```python
from build123d import *

# Parameters (mm, degrees)
SKETCH_1_W                      = 7.778385112
SKETCH_1_H                      = 31.92137072
EXTRUDE_1_DEPTH                 = 8
SKETCH_2_R                      = 1.5
SKETCH_2_R_2                    = 2
CUT_EXTRUDE_1_DEPTH             = 8
SKETCH_3_W                      = 7.778385112
SKETCH_3_H                      = 11.681320089
CUT_EXTRUDE_2_DEPTH             = 7
CUT_EXTRUDE_3_DEPTH             = 7.778385113
CUT_EXTRUDE_6_REACH             = 24.375
CUT_EXTRUDE_7_DEPTH             = 1.25
CUT_EXTRUDE_7_DEPTH_BACK        = 1.25
CUT_EXTRUDE_8_REACH             = 24.375
SKETCH_8_R                      = 1
PATTERN_CIRCULAR_5_COUNT        = 2
CUT_EXTRUDE_9_DEPTH             = 23.991982407
CUT_EXTRUDE_9_DEPTH_BACK        = 23.991982407
PATTERN_START                   = 3.938890695
PATTERN_CIRCULAR_14_OUTLINE_R   = 1
PATTERN_CIRCULAR_14_DEPTH       = 3.518451758
PATTERN_START_2                 = 9.957342453
PATTERN_CIRCULAR_14_2_OUTLINE_R = 1
PATTERN_CIRCULAR_14_2_DEPTH     = 1.78640085


# Read off the part's stored shape, not the designer's step: 阵列(圆周)14
with BuildPart() as part:
    # 草图1 → 凸台-拉伸1 (new body)
    with BuildSketch(Plane(origin=(0, 0, 0), x_dir=(1, 0, 0), z_dir=(0, 1, 0))):
        Rectangle(SKETCH_1_W, SKETCH_1_H)
    extrude(amount=EXTRUDE_1_DEPTH)

    # 草图2 → 切除-拉伸1 (cut)
    with BuildSketch(Plane(origin=(0, 8, 0), x_dir=(1, 0, 0), z_dir=(0, 1, 0))):
        with Locations(Location((0, 6, 0), (0, 0, 270))):
            Circle(SKETCH_2_R)
        with Locations(Location((0, -6, 0), (0, 0, 270))):
            Circle(SKETCH_2_R)
        with Locations(Location((0, 0, 0), (0, 0, 270))):
            Circle(SKETCH_2_R_2)
    extrude(amount=-CUT_EXTRUDE_1_DEPTH, mode=Mode.SUBTRACT)

    # 草图3 → 切除-拉伸2 (cut)
    with BuildSketch(Plane(origin=(0, 6.911179492, -11.97051402), x_dir=(-1, 0, 0), z_dir=(0, -0.499999999999998, 0.8660254037844398))):
        with Locations((0, 2.139682636)):
            Rectangle(SKETCH_3_W, SKETCH_3_H)
    cut_extrude_2 = extrude(amount=-CUT_EXTRUDE_2_DEPTH, mode=Mode.SUBTRACT)

    # 草图4 → 切除-拉伸3 (cut)
    with BuildSketch(Plane.ZY.offset(3.889192556)):
        Polygon((-14.378284056, 2.740799456), (-9.631080146, 0), (-15.96068536, 0), align=None)
    cut_extrude_3 = extrude(amount=-CUT_EXTRUDE_3_DEPTH, mode=Mode.SUBTRACT)

    # 切除-拉伸6: up to this plane
    cut_extrude_6_end = Plane(origin=(0, 8, 0), z_dir=(0, 1, 0))
    # 草图6 → 切除-拉伸6 (cut, up to the surface)
    with BuildSketch(Plane(origin=(0, -4.170380036, -2.407770036), x_dir=(1, 0, 0), z_dir=(0, -0.8660254037844396, -0.4999999999999982)), mode=Mode.PRIVATE) as cut_extrude_6_sk1:
        with BuildLine():
            Line((-3.889192556, -13.822358983), (5e-09, -13.822358983))
            ThreePointArc((5e-09, -13.822358983), (-2.384323859, -13.062439969), (-3.889192556, -11.062978192))
            Line((-3.889192556, -11.062978192), (-3.889192556, -13.822358983))
        make_face()
    cut_extrude_6_tool1 = split(extrude(cut_extrude_6_sk1.sketch, amount=-CUT_EXTRUDE_6_REACH, mode=Mode.PRIVATE), bisect_by=cut_extrude_6_end, keep=Keep.BOTH, mode=Mode.PRIVATE)
    add(cut_extrude_6_tool1.solids().sort_by_distance((-2.992661, 2.37004, -13.736111))[0], mode=Mode.SUBTRACT)
    # 草图6 → 切除-拉伸6 (cut, up to the surface)
    with BuildSketch(Plane(origin=(0, -4.170380036, -2.407770036), x_dir=(1, 0, 0), z_dir=(0, -0.8660254037844396, -0.4999999999999982)), mode=Mode.PRIVATE) as cut_extrude_6_sk2:
        with BuildLine():
            Line((3.889192556, -13.822358983), (3.889192556, -11.062978192))
            ThreePointArc((3.889192556, -11.062978192), (2.384323863, -13.062439966), (5e-09, -13.822358983))
            Line((5e-09, -13.822358983), (3.889192556, -13.822358983))
        make_face()
    cut_extrude_6_tool2 = split(extrude(cut_extrude_6_sk2.sketch, amount=-CUT_EXTRUDE_6_REACH, mode=Mode.PRIVATE), bisect_by=cut_extrude_6_end, keep=Keep.BOTH, mode=Mode.PRIVATE)
    add(cut_extrude_6_tool2.solids().sort_by_distance((2.992661, 2.37004, -13.736111))[0], mode=Mode.SUBTRACT)

    # 草图7 → 切除-拉伸7 (cut, two sides: drawn at the far end of the back side and taken through both)
    with BuildSketch(Plane(origin=(0, -1.540779764, -0.889569611), x_dir=(-1, 0, 0), z_dir=(0, -0.8660254037844396, -0.4999999999999983)).offset(-CUT_EXTRUDE_7_DEPTH_BACK)):
        with BuildLine():
            Line((-3.889192556, 11.062978192), (-3.889192556, 8.340760072))
            Line((-3.889192556, 8.340760072), (3.889192556, 8.340760072))
            Line((3.889192556, 8.340760072), (3.889192556, 11.062978192))
            ThreePointArc((3.889192556, 11.062978192), (0, 13.822358983), (-3.889192556, 11.062978192))
        make_face()
    extrude(amount=CUT_EXTRUDE_7_DEPTH + CUT_EXTRUDE_7_DEPTH_BACK, mode=Mode.SUBTRACT)

    # 切除-拉伸8: up to this plane
    cut_extrude_8_end = Plane(origin=(0, 8, 0), z_dir=(0, 1, 0))
    # 草图8 → 切除-拉伸8 (cut, up to the surface)
    with BuildSketch(Plane(origin=(0, -4.170380036, -2.407770036), x_dir=(1, 0, 0), z_dir=(0, -0.8660254037844396, -0.4999999999999982)), mode=Mode.PRIVATE) as cut_extrude_8_sk1:
        with Locations(Location((0, -11.822358983, 0), (0, 0, 270))):
            Circle(SKETCH_8_R)
    cut_extrude_8_tool1 = split(extrude(cut_extrude_8_sk1.sketch, amount=-CUT_EXTRUDE_8_REACH, mode=Mode.PRIVATE), bisect_by=cut_extrude_8_end, keep=Keep.BOTH, mode=Mode.PRIVATE)
    add(cut_extrude_8_tool1.solids().sort_by_distance((0, 1.740799, -12.646233))[0], mode=Mode.SUBTRACT)

    # 阵列(圆周)5: 切除-拉伸2, 切除-拉伸3 ×2 about axis
    pattern_circular_5_axis = Axis((-4.278111812, 4, 0), (1, 0, 0))
    add([cut_extrude_2.rotate(pattern_circular_5_axis, i * 360 / PATTERN_CIRCULAR_5_COUNT) for i in range(1, PATTERN_CIRCULAR_5_COUNT)], mode=Mode.SUBTRACT)
    add([cut_extrude_3.rotate(pattern_circular_5_axis, i * 360 / PATTERN_CIRCULAR_5_COUNT) for i in range(1, PATTERN_CIRCULAR_5_COUNT)], mode=Mode.SUBTRACT)

    # 草图10 → 切除-拉伸9 (cut, two sides: drawn at the far end of the back side and taken through both)
    with BuildSketch(Plane(origin=(0, 10.170380036, 5.871871652), x_dir=(1, 0, 0), z_dir=(0, 0.8660254037844388, 0.49999999999999994)).offset(-CUT_EXTRUDE_9_DEPTH_BACK)):
        with BuildLine():
            ThreePointArc((0, -9.822358983), (-2.384323861, -9.062439968), (-3.889192556, -7.062978192))
            Line((-3.889192556, -7.062978192), (-3.889192556, -9.822358983))
            Line((-3.889192556, -9.822358983), (0, -9.822358983))
        make_face()
        with BuildLine():
            ThreePointArc((3.889192556, -7.062978192), (2.384323861, -9.062439968), (0, -9.822358983))
            Line((0, -9.822358983), (3.889192556, -9.822358983))
            Line((3.889192556, -9.822358983), (3.889192556, -7.062978192))
        make_face()
    extrude(amount=CUT_EXTRUDE_9_DEPTH + CUT_EXTRUDE_9_DEPTH_BACK, mode=Mode.SUBTRACT)

    # 阵列(圆周)14 outline → 阵列(圆周)14 (cut)
    with BuildSketch(Plane(origin=(0, 0, 0), x_dir=(1, 0, 0), z_dir=(0, 0.8660254037844399, 0.49999999999999795)).offset(PATTERN_START)):
        with Locations((0, -7.822358983)):
            Circle(PATTERN_CIRCULAR_14_OUTLINE_R)
    extrude(amount=PATTERN_CIRCULAR_14_DEPTH, mode=Mode.SUBTRACT)

    # Pattern Circular 14 2 outline → Pattern Circular 14 2 (cut)
    with BuildSketch(Plane(origin=(0, 0, 0), x_dir=(1, 0, 0), z_dir=(0, 0.8660254037844399, 0.49999999999999795)).offset(PATTERN_START_2)):
        with Locations((0, -7.822358983)):
            Circle(PATTERN_CIRCULAR_14_2_OUTLINE_R)
    extrude(amount=PATTERN_CIRCULAR_14_2_DEPTH, mode=Mode.SUBTRACT)


solid = part.part
```
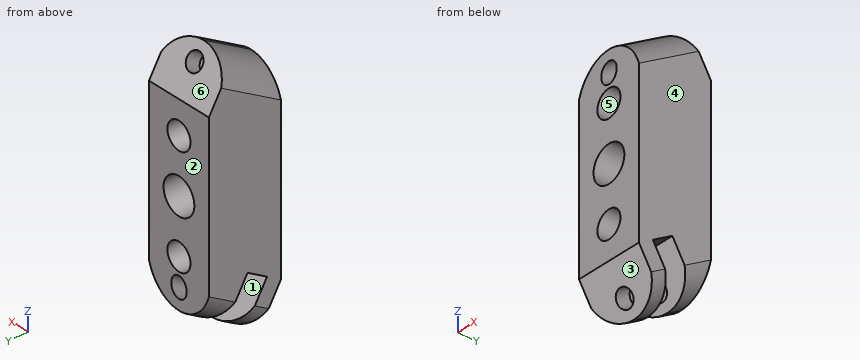
CAD build for the part. Positions are in the model's coordinates, mm. Face numbers are marked on the shaded views. A direction names the side the tool comes from. Round coordinates to 2 decimals unless told otherwise and drop trailing zeros. Order: outer loops, then holes, each group sorted by start corner. A loop starts at its lowest first (then second) coordinate and runs counter-clockwise, first axis right, second up.
Item 1: Probe line 1 along X through (y, z) = (3.75, 0); line 2 along X through (y, z) = (6, -6); line 3 along Z through (x, y) = (0.75, 4.75). List the from-to ranges inside material, lowest first.
Item 2: Tool access for the marked faces 1 and 2: list every direction of +Z, -Z, +X, -X, +Y, -Y with a clear straight run to the whole face (end or side of a thin tool).
Item 3: Pin check, flat tips, straight feed: pin 1 (1.5 mm diameter, centred on x = -1, y = 3, fed in from +Z); pin 2 (2 mm diameter, centred on y = 1, z = 10.5, fed in from +X). Stop position of each tip, or through.
Item 4: Mould opens along Z. For the marked faces 3, 4, 5 and 6 say: pulls with the +Z half, pulls with the -Z half, needs draft (parallel to the pull), parting line crosses it, or undercut.
Item 5: Saw through at C-C on x = -0.5. State how many separate pieces and enclosed holes the cut face has, then the cut area to 3 significant figures.
Item 6: Saw through at A-A on z = 0. Write the cut outline in (x, y), then the cut area to 3 significant figures.
Item 7: Saw through at B-B on z = -6. Write the cut outline in (x, y).
Reported:
1. line 1: x = -3.89 to -2, 2 to 3.89
1. line 2: x = -3.89 to -1.5, 1.5 to 3.89
1. line 3: z = -9.29 to -7.3, -4.7 to -1.85, 1.85 to 4.7, 7.3 to 11.69, 12.54 to 14
2. face 1: +X, -X
2. face 2: +Z, -Z, +X, -X, +Y
3. pin 1: stops at z = 13.4
3. pin 2: stops at x = 3.66
4. face 3: pulls with the -Z half
4. face 4: needs draft
4. face 5: undercut
4. face 6: pulls with the +Z half
5. separate pieces: 6
5. enclosed holes: 0
5. area: 94.5 mm2
6. outline: (-3.89, 0) - (-2, 0) - (-2, 8) - (-3.89, 8) - close; (2, 0) - (3.89, 0) - (3.89, 8) - (2, 8) - close
6. area: 30.2 mm2
7. outline: (-3.89, 0) - (-1.5, 0) - (-1.5, 8) - (-3.89, 8) - close; (1.5, 0) - (3.89, 0) - (3.89, 8) - (1.5, 8) - close
